Check sheet for the modelled part. Datum: model origin and axes. Units: mm. Round coordinates to 2 decimals unless told otherwise and drop trailing zeros. Use CSV: the item, a comma, the result in double quotes.
```python
from build123d import *

# Parameters (mm, degrees)
SKETCH6_W      = 16.950500326
SKETCH6_H      = 13.781908613
EXTRUDE1_DEPTH = 3.99736
FILLET1_R      = 1.27


with BuildPart() as part:
    # Sketch1 → Revolve1 (revolve)
    with BuildSketch(Plane.XY):
        Polygon((0, 0), (0, 5.446572654), (0.025429996, 5.493979528), (0.64160868, 6.642666473), (0.695379235, 6.644346887), (1.382081969, 5.53637702), (1.435852524, 5.538057434), (2.052031208, 6.686744379), (2.105801763, 6.688424793), (2.792504496, 5.580454927), (2.846275051, 5.582135341), (3.462453735, 6.730822286), (3.51622429, 6.7325027), (4.202927024, 5.624532834), (4.256697579, 5.626213248), (4.872876263, 6.774900193), (4.926646818, 6.776580606), (5.613349551, 5.66861074), (5.667120106, 5.670291154), (6.28329879, 6.818978099), (6.337069345, 6.820658513), (7.023772079, 5.712688647), (7.077542634, 5.714369061), (7.693721318, 6.863056006), (7.747491873, 6.86473642), (8.434194606, 5.756766554), (8.487965161, 5.758446968), (9.104143845, 6.907133913), (9.1579144, 6.908814326), (9.844617134, 5.80084446), (9.898387689, 5.802524874), (10.514566373, 6.951211819), (10.568336928, 6.952892233), (11.255039661, 5.844922367), (11.308810216, 5.846602781), (11.9249889, 6.995289726), (11.978759455, 6.99697014), (12.665462189, 5.889000274), (12.719232744, 5.890680687), (13.335411428, 7.039367633), (13.389181983, 7.041048046), (14.075884716, 5.93307818), (14.129655271, 5.934758594), (14.745833955, 7.083445539), (14.79960451, 7.085125953), (15.486307244, 5.977156087), (15.540077799, 5.978836501), (16.156256483, 7.127523446), (16.210027038, 7.12920386), (16.896729771, 6.021233994), (16.950500326, 6.022914407), (16.950500326, 0), align=None)
    revolve(axis=Axis((0, 0, 0), (-1, 0, 0)))

    # Sketch5 → Cut-Revolve2 (revolve, cut)
    with BuildSketch(Plane.XY):
        Polygon((15.10284, 0), (15.10284, 7.094602536), (16.950500326, 7.152344806), (16.950500326, 0), align=None)
    revolve(axis=Axis((0, 0, 0), (-1, 0, 0)), mode=Mode.SUBTRACT)

    # Sketch6 → Cut-Revolve3 (revolve, cut)
    with BuildSketch(Plane.XY):
        with Locations((8.475250163, 13.748954307)):
            Rectangle(SKETCH6_W, SKETCH6_H)
    revolve(axis=Axis((0, 0, 0), (1, 0, 0)), mode=Mode.SUBTRACT)

    # Sketch7 → Revolve2 (revolve)
    with BuildSketch(Plane.XY):
        Polygon((10.2108, 5.446572654), (15.10284, 6.858), (15.10284, 5.446572654), align=None)
    revolve(axis=Axis((0, 0, 0), (1, 0, 0)))

    # Sketch8 → Extrude1 (add)
    with BuildSketch(Plane(origin=(15.10284, 0, 0), x_dir=(0, 0, -1), z_dir=(1, 0, 0))):
        Polygon((0, 8.212230229), (-7.112, 4.106115114), (-7.112, -4.106115114), (0, -8.212230229), (7.112, -4.106115114), (7.112, 4.106115114), align=None)
    extrude(amount=EXTRUDE1_DEPTH)

    # Sketch9 → Cut-Revolve4 (revolve, cut)
    with BuildSketch(Plane.XY):
        Polygon((19.1002, 6.942230229), (18.626431419, 7.958230229), (15.576608581, 7.958230229), (15.10284, 6.942230229), (15.10284, 8.212230229), (19.1002, 8.212230229), align=None)
    revolve(axis=Axis((0, 0, 0), (1, 0, 0)), mode=Mode.SUBTRACT)

    # Sketch10 → Revolve3 (revolve)
    with BuildSketch(Plane.XY):
        with BuildLine():
            Line((19.1002, 0), (42.9, 0))
            Line((42.9, 0), (42.9, 3.96875))
            Line((42.9, 3.96875), (38.1375, 3.96875))
            Line((38.1375, 3.96875), (36.362408616, 5.458228526))
            Line((36.362408616, 5.458228526), (35.092408616, 5.458228526))
            Line((35.092408616, 5.458228526), (33.317317232, 3.96875))
            Line((33.317317232, 3.96875), (31.0001, 3.96875))
            Line((31.0001, 3.96875), (28.619597791, 5.966228526))
            Line((28.619597791, 5.966228526), (26.302380559, 5.966228526))
            Line((26.302380559, 5.966228526), (26.302380559, 5.712228526))
            Line((26.302380559, 5.712228526), (22.6562, 5.712228526))
            Line((22.6562, 5.712228526), (22.6562, 5.966228526))
            Line((22.6562, 5.966228526), (21.3862, 5.966228526))
            ThreePointArc((21.3862, 5.966228526), (20.8782, 5.712228526), (20.3702, 5.966228526))
            Line((20.3702, 5.966228526), (19.1002, 5.966228526))
            Line((19.1002, 5.966228526), (19.1002, 0))
        make_face()
    revolve(axis=Axis((0, 0, 0), (-1, 0, 0)))

    # Fillet1
    fillet1_edges = [part.edges().sort_by_distance(p)[0] for p in [
        (42.9, -3.96875, 0),
    ]]
    fillet(fillet1_edges, radius=FILLET1_R)

    # Sketch11 → Cut-Revolve5 (revolve, cut)
    with BuildSketch(Plane.XY):
        Polygon((15.10284, 4.6228), (19.1002, 1.984375), (42.9, 1.984375), (42.9, 0), (10.2108, 0), (0, 0), (0, 4.6228), align=None)
    revolve(axis=Axis((0, 0, 0), (-1, 0, 0)), mode=Mode.SUBTRACT)


solid = part.part
```
Q1. Scan lines: L1, parallel to Y at x = 5.5, z = 0; L2, parallel to Z at x = 12, y = 0; L3, parallel to Y at x = 36, z = 0. Record each from-to range of solid material in increasing order.
Result sheet:
L1,"y = -5.85 to -4.62, 4.62 to 5.85"
L2,"z = -6.86 to -4.62, 4.62 to 6.86"
L3,"y = -5.46 to -1.98, 1.98 to 5.46"
Q2. Go/stop test with flat-tipped pins: pin 1 (2 mm diameter, centred on x = 18, y = -5, fed in from +Z); pin 2 (7 mm diameter, centred on y = 0, z = 1, fed in from -X); pin 3 (3 mm diameter, centred on y = 2.5, z = 1, fed in from -X); pin 4 (3 mm diameter, centred on y = 0, z = 0, fed in from +X). Record where each tip stops, or that it passes through.
Result sheet:
pin 1,"stops at z = 6.88"
pin 2,"stops at x = 15.29"
pin 3,"stops at x = 15.75"
pin 4,"passes through"
Q3. Mould release check, pull along X, two halves, no side actions. Record for faces 1 (the face through (32.142, -0.86, 3.874)), 2 (the face through (14.78, 6.54, 2.06)): pulls with the +X half, pulls with the -X half, needs draft (parallel to the pull), parting line crosses it, or undercut.
Result sheet:
face 1,"undercut"
face 2,"needs draft"
